The listing builds one solid part. Answer for the finished solid, in the listing's coordinates (mm). Face numbers are marked on the shaded views. A direction names the side the tool comes from. Coordinates: 2 decimals unless noted, no trailing zeros. Order: outer loops, then holes, each group sorted by start corner. A loop starts at its lowest first (then second) coordinate and runs counter-clockwise, first axis right, second up.
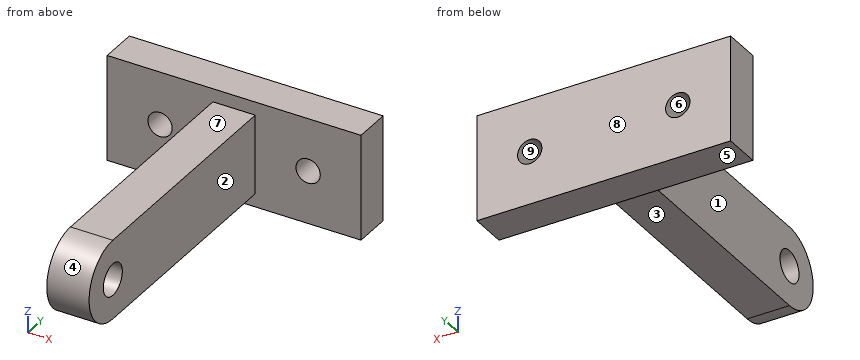
Autodesk Inventor part; units mm, degrees
ref_plane "YZ Plane" through (0, 0, 0) normal (1, 0, 0) x (0, 1, 0)
ref_plane "XZ Plane" through (0, 0, 0) normal (0, 1, 0) x (-1, 0, 0)
ref_plane "XY Plane" through (0, 0, 0) normal (0, 0, 1) x (1, 0, 0)
sketch "Sketch1" plane through (0, 0, 0) normal (1, 0, 0) x (0, 1, 0)
  circle A0 centre (0, 0) radius 3
  circle A1 centre (0, 0) radius 7.5
  line L0 (0, 7.5) -> (45, 7.5)
  line L1 (45, 7.5) -> (45, -7.5)
  line L2 (45, -7.5) -> (0, -7.5)
  dimension "d0" = 6
  dimension "d1" = 15
  dimension "d2" = 45
extrude "Extrusion1" add sketch "Sketch1" along normal blind 8
sketch "Sketch2" plane through (0, 0, 0) normal (-1, 0, 0) x (0, 0, 1)
  line L0 (-10, 45) -> (10, 45)
  line L1 (10, 45) -> (10, 52)
  line L2 (10, 52) -> (-10, 52)
  line L3 (-10, 52) -> (-10, 45)
  line L4 (7.5, 45) -> (7.5, 0)
  line L5 (-7.5, 45) -> (7.5, 45)
  point P0 (0, 0)
  dimension "d5" = 20
  dimension "d6" = 2.5
  dimension "d7" = 0
  dimension "d8" = 7
extrude "Extrusion2" add sketch "Sketch2" along normal blind 20 and the other way blind 28
sketch "Sketch3" plane through (-20, 45, 10) normal (0, -1, 0) x (1, 0, 0)
  circle A0 centre (38, -10) radius 2.3
  circle A1 centre (10, -10) radius 2.3
  line L0 (48, 0) -> (0, 0)
  line L1 (48, 0) -> (48, -20)
  line L2 (0, -20) -> (0, 0)
  point P0 (20, -10)
  dimension "d13" = 10
  dimension "d14" = 10
  dimension "d15" = 4.6
  dimension "d16" = 4.6
  dimension "d17" = 10
  dimension "d18" = 10
extrude "Extrusion3" cut sketch "Sketch3" against normal mid plane 20
equation "\"d14\" = d13"
equation "\"d15\" = d16"
equation "\"d17\" = d14"
equation "\"d18\" = d13"
properties part number "RouleauMount"
(1) Find section A-A (x = 18). Write down the section's boundary in (y, z).
(2) The mould has two halves that part along Z. Classify the marked faces 6, 7, 8 and 9: released by +Z, released by -Z, zero draft, split by the parting line, or undercut.
(3) Find section C-C (x = 3). Write down the section's boundary in (y, z).
(4) Find section B-B (z = 0). Write down the section's boundary in (x, y).
(5) Consider line 1 (Z direction, x = -10, y = 47); line 2 (Z direction, x = 6, y = 0); line 3 (X direction, y = 4, z = 4). Determine where each line is inside the solid, lowest interval first.
(6) Find section D-D (z = 5.75). Write down the section's boundary in (x, y).
(7) Each of these flat-tipped pins is pushed along its axis until it touches: pin 1 Ø7 at (y, z) = (0, 0) entering from -X; pin 2 Ø12 at (y, z) = (20, 1) entering from +X; pin 3 Ø2.5 at (x, y) = (5.5, 20.5) entering from -Z; pin 4 Ø10 at (x, y) = (-7.5, 16) entering from -Z. Where does it stop, or does it pass through?
(8) For the marked faces 1, 2, 3, 4 and 5, determine the directions among +Z, -Z, +X, -X, +Y, -Y from which every point of the face is accessible in a straight line to the end or side of a thin tool.
Findings below:
1. outline: (45, -10) - (52, -10) - (52, -2.3) - (45, -2.3) - close; (45, 2.3) - (52, 2.3) - (52, 10) - (45, 10) - close
2. face 6: undercut
2. face 7: released by +Z
2. face 8: zero draft
2. face 9: undercut
3. outline: (0, -7.5) - (45, -7.5) - (45, -10) - (52, -10) - (52, 10) - (45, 10) - (45, 7.5) - (0, 7.5) arc R7.5 ccw to start; hole circle Ø6 at (0, 0)
4. outline: (-20, 45) - (-12.3, 45) - (-12.3, 52) - (-20, 52) - close; (-7.7, 45) - (0, 45) - (0, 3) - (8, 3) - (8, 45) - (15.7, 45) - (15.7, 52) - (-7.7, 52) - close; (0, -7.5) - (8, -7.5) - (8, -3) - (0, -3) - close; (20.3, 45) - (28, 45) - (28, 52) - (20.3, 52) - close
5. line 1: z = -10 to -2.3, 2.3 to 10
5. line 2: z = -7.5 to -3, 3 to 7.5
5. line 3: x = 0 to 8
6. outline: (-20, 45) - (0, 45) - (0, -4.82) - (8, -4.82) - (8, 45) - (28, 45) - (28, 52) - (-20, 52) - close
7. pin 1: stops at x = 0
7. pin 2: stops at x = 8
7. pin 3: stops at z = -7.5
7. pin 4: passes through
8. face 1: +Z, -Z, -X, -Y
8. face 2: +Z, -Z, +X, -Y
8. face 3: -Z, +X, -X, -Y
8. face 4: +X, -X, -Y
8. face 5: -Z, +X, -X, +Y, -Y
